```python
from build123d import *

# Parameters (mm, degrees)
SKETCH_1_W          = 100
SKETCH_1_H          = 44
EXTRUDE_1_DEPTH     = 21
CHAMFER_1_SIZE      = 5
SKETCH_2_R          = 3
CUT_EXTRUDE_1_DEPTH = 112.251966275
SKETCH_3_W          = 9
SKETCH_3_H          = 9
CUT_EXTRUDE_2_DEPTH = 9.5
SKETCH_4_R          = 18
CUT_EXTRUDE_3_DEPTH = 2
SKETCH_5_W          = 10
SKETCH_5_H          = 10
CUT_EXTRUDE_4_DEPTH = 9
FILLET_1_R          = 7


with BuildPart() as part:
    # 草图1 → 凸台-拉伸1 (new body)
    with BuildSketch(Plane(origin=(0, 0, 0), x_dir=(1, 0, 0), z_dir=(0, 1, 0))):
        with Locations((50, 22)):
            Rectangle(SKETCH_1_W, SKETCH_1_H)
    extrude(amount=EXTRUDE_1_DEPTH)

    # 倒角1
    chamfer_1_edges = [part.edges().sort_by_distance(p)[0] for p in [
        (50, 0, -44),
        (50, 0, 0),
    ]]
    chamfer(chamfer_1_edges, length=CHAMFER_1_SIZE)

    # 草图2 → 切除-拉伸1 (cut, through all)
    with BuildSketch(Plane(origin=(0, 21, 0), x_dir=(1, 0, 0), z_dir=(0, 1, 0))):
        with Locations(Location((96, 4, 0), (0, 0, 270))):
            Circle(SKETCH_2_R)
        with Locations(Location((4, 4, 0), (0, 0, 160.528779366))):
            Circle(SKETCH_2_R)
        with Locations(Location((4, 40, 0), (0, 0, 270))):
            Circle(SKETCH_2_R)
        with Locations(Location((96, 40, 0), (0, 0, 199.471220634))):
            Circle(SKETCH_2_R)
    extrude(amount=-CUT_EXTRUDE_1_DEPTH, mode=Mode.SUBTRACT)

    # 草图3 → 切除-拉伸2 (cut)
    with BuildSketch(Plane(origin=(0, 21, 0), x_dir=(1, 0, 0), z_dir=(0, 1, 0))):
        with Locations((95.5, 4.5)):
            Rectangle(SKETCH_3_W, SKETCH_3_H)
        with Locations((4.5, 4.5)):
            Rectangle(SKETCH_3_W, SKETCH_3_H)
        with Locations((95.5, 39.5)):
            Rectangle(SKETCH_3_W, SKETCH_3_H)
        with Locations((4.5, 39.5)):
            Rectangle(SKETCH_3_W, SKETCH_3_H)
    extrude(amount=-CUT_EXTRUDE_2_DEPTH, mode=Mode.SUBTRACT)

    # 草图4 → 切除-拉伸3 (cut)
    with BuildSketch(Plane(origin=(0, 21, 0), x_dir=(1, 0, 0), z_dir=(0, 1, 0))):
        with Locations(Location((28.5, 22, 0), (0, 0, 270))):
            Circle(SKETCH_4_R)
        with Locations(Location((71.5, 22, 0), (0, 0, 90))):
            Circle(SKETCH_4_R)
    extrude(amount=-CUT_EXTRUDE_3_DEPTH, mode=Mode.SUBTRACT)

    # 草图5 → 切除-拉伸4 (cut)
    with BuildSketch(Plane.XZ):
        with Locations((95, -39)):
            Rectangle(SKETCH_5_W, SKETCH_5_H)
        with Locations((95, -5)):
            Rectangle(SKETCH_5_W, SKETCH_5_H)
        with Locations((5, -5)):
            Rectangle(SKETCH_5_W, SKETCH_5_H)
        with Locations((5, -39)):
            Rectangle(SKETCH_5_W, SKETCH_5_H)
    extrude(amount=-CUT_EXTRUDE_4_DEPTH, mode=Mode.SUBTRACT)

    # 圆角1
    # the kernel refuses this fillet: 7 mm, written as the material it adds along each edge
    with BuildSketch(Plane(origin=(9, 21, -35), x_dir=(-1, 0, 0), z_dir=(0, -1, 0))) as fillet_1_piece_1:
        with BuildLine():
            CenterArc((FILLET_1_R, FILLET_1_R), FILLET_1_R, 180, 90)
            Line((0, FILLET_1_R), (0, 0))
            Line((0, 0), (FILLET_1_R, 0))
        make_face()
    extrude(amount=9.5)
    with BuildSketch(Plane(origin=(9, 21, -9), x_dir=(0, 0, 1), z_dir=(0, -1, 0))) as fillet_1_piece_2_section:
        with BuildLine():
            CenterArc((FILLET_1_R, FILLET_1_R), FILLET_1_R, 180, 90)
            Line((0, FILLET_1_R), (0, 0))
            Line((0, 0), (FILLET_1_R, 0))
        make_face()
    fillet_1_piece_2 = extrude(amount=27, mode=Mode.PRIVATE)
    fillet_1_piece_2 = split(fillet_1_piece_2, bisect_by=Plane(origin=(7.436424427, 9, -7.436424427), z_dir=(0, 1, 0)), keep=Keep.TOP, mode=Mode.PRIVATE)
    add(fillet_1_piece_2)
    with BuildSketch(Plane(origin=(10, 0, -10), x_dir=(0, 0, 1), z_dir=(0, 1, 0))) as fillet_1_piece_3_section:
        with BuildLine():
            CenterArc((FILLET_1_R, -FILLET_1_R), FILLET_1_R, 90, 90)
            Line((0, -FILLET_1_R), (0, 0))
            Line((0, 0), (FILLET_1_R, 0))
        make_face()
    fillet_1_piece_3 = extrude(amount=26.5, mode=Mode.PRIVATE)
    fillet_1_piece_3 = split(fillet_1_piece_3, bisect_by=Plane(origin=(9.565673238, 1.191688147, -3.808311853), z_dir=(0, 0.7071067811865476, -0.7071067811865476)), keep=Keep.TOP, mode=Mode.PRIVATE)
    fillet_1_piece_3 = split(fillet_1_piece_3, bisect_by=Plane(origin=(9.565673238, 21, -7.128953399), z_dir=(0, -1, 0)), keep=Keep.TOP, mode=Mode.PRIVATE)
    add(fillet_1_piece_3)
    with BuildSketch(Plane(origin=(10, 0, -34), x_dir=(-1, 0, 0), z_dir=(0, 1, 0))) as fillet_1_piece_4_section:
        with BuildLine():
            CenterArc((FILLET_1_R, -FILLET_1_R), FILLET_1_R, 90, 90)
            Line((0, -FILLET_1_R), (0, 0))
            Line((0, 0), (FILLET_1_R, 0))
        make_face()
    fillet_1_piece_4 = extrude(amount=26.5, mode=Mode.PRIVATE)
    fillet_1_piece_4 = split(fillet_1_piece_4, bisect_by=Plane(origin=(7.120179523, 21, -34.433198562), z_dir=(0, -1, 0)), keep=Keep.TOP, mode=Mode.PRIVATE)
    fillet_1_piece_4 = split(fillet_1_piece_4, bisect_by=Plane(origin=(7.120179523, -0.033400719, -38.966599281), z_dir=(0, 0.7071067811865476, 0.7071067811865476)), keep=Keep.TOP, mode=Mode.PRIVATE)
    add(fillet_1_piece_4)
    with BuildSketch(Plane(origin=(91, 21, -35), x_dir=(1, 0, 0), z_dir=(0, -1, 0)), Plane(origin=(91, 21, -9), x_dir=(0, 0, 1), z_dir=(0, -1, 0))) as fillet_1_piece_5:
        with BuildLine():
            CenterArc((FILLET_1_R, -FILLET_1_R), FILLET_1_R, 90, 90)
            Line((0, -FILLET_1_R), (0, 0))
            Line((0, 0), (FILLET_1_R, 0))
        make_face()
    extrude(amount=9.5)
    with BuildSketch(Plane(origin=(90, 0, -34), x_dir=(1, 0, 0), z_dir=(0, 1, 0))) as fillet_1_piece_6_section:
        with BuildLine():
            CenterArc((FILLET_1_R, FILLET_1_R), FILLET_1_R, 180, 90)
            Line((0, FILLET_1_R), (0, 0))
            Line((0, 0), (FILLET_1_R, 0))
        make_face()
    fillet_1_piece_6 = extrude(amount=26.5, mode=Mode.PRIVATE)
    fillet_1_piece_6 = split(fillet_1_piece_6, bisect_by=Plane(origin=(92.879820477, 21, -34.433198562), z_dir=(0, -1, 0)), keep=Keep.TOP, mode=Mode.PRIVATE)
    fillet_1_piece_6 = split(fillet_1_piece_6, bisect_by=Plane(origin=(92.879820477, -0.033400719, -38.966599281), z_dir=(0, 0.7071067811865476, 0.7071067811865476)), keep=Keep.TOP, mode=Mode.PRIVATE)
    add(fillet_1_piece_6)
    with BuildSketch(Plane(origin=(90, 0, -10), x_dir=(0, 0, 1), z_dir=(0, 1, 0))) as fillet_1_piece_7_section:
        with BuildLine():
            CenterArc((FILLET_1_R, FILLET_1_R), FILLET_1_R, 180, 90)
            Line((0, FILLET_1_R), (0, 0))
            Line((0, 0), (FILLET_1_R, 0))
        make_face()
    fillet_1_piece_7 = extrude(amount=26.5, mode=Mode.PRIVATE)
    fillet_1_piece_7 = split(fillet_1_piece_7, bisect_by=Plane(origin=(90.434326762, 1.191688147, -3.808311853), z_dir=(0, 0.7071067811865476, -0.7071067811865476)), keep=Keep.TOP, mode=Mode.PRIVATE)
    fillet_1_piece_7 = split(fillet_1_piece_7, bisect_by=Plane(origin=(90.434326762, 21, -7.128953399), z_dir=(0, -1, 0)), keep=Keep.TOP, mode=Mode.PRIVATE)
    add(fillet_1_piece_7)


solid = part.part
```
Read the model definition and answer for the solid it produces. Units are mm, in the model's axes. A direction names the side the tool comes from. Give positions to 0.01 mm unless a question says otherwise; leave off trailing zeros. Order: outer loops, then holes, each group sorted by start corner. A loop starts at its lowest first (then second) coordinate and runs counter-clockwise, first axis right, second up.
(1) For faces 1 (the flat face through (1, 16, -35)), 2 (the flat face through (93, 9, -5)), 3 (the flat face through (5, 9, -7)), 4 (the cylindrical face through (92, 4.4, -36.1)), 5 (the flat face through (99, 16, -9)), determine the directions among +Z, -Z, +X, -X, +Y, -Y from which every point of the face is accessible in a straight line to the end or side of a thin tool.
(2) Given pin 1 (0.6 mm diameter, centred on y = 14, z = -42.5, fed in from -X); pin 2 (7 mm diameter, centred on x = 97, z = -3.5, fed in from +Y); pin 3 (0.9 mm diameter, centred on y = 7, z = -2, fed in from +X), each flat-ended and moving along its own axis, determine where each tip first touches the part or whether it passes through.
(3) Find section D-D (x = 96). Give the vertices of the cut face in (y, z).
(4) Find section B-B (x = 28.5). Give the vertices of the cut face in (y, z), plus the area to 3 significant figures.
(5) For a pull along Z with two mould halves and no side action, classify faces 6 (the flat face through (29, 19, -22)), 7 (the flat face through (1, 4, -34)), 8 (the flat face through (10, 6, -43)) as released by +Z, released by -Z, zero draft, split by the parting line, or undercut.
(6) Straight lines are drawn through the part: L1, parallel to X at y = 10.45, z = -4; L2, parallel to X at y = 19.55, z = -22; L3, parallel to Z at x = 71.5, y = 20.15. For each, find the intervals that lie inside material, in ascending order.
(7) Find section A-A (z = -22). Give the vertices of the cut face in (x, y).
(8) Find section C-C (y = 6). Give the vertices of the cut face in (x, z), plus the area to 3 significant figures.
Result sheet:
1. face 1: -Z, -X, +Y
1. face 2: +Z, +X, -Y
1. face 3: +Z, -X, -Y
1. face 4: -Z, +X, -Y
1. face 5: +Z, +X, +Y
2. pin 1: stops at x = 9
2. pin 2: stops at y = 11.5
2. pin 3: stops at x = 90
3. outline: (0, -34.07) - (9, -34.07) - (9, -37) - (11.5, -37) - (11.5, -35.29) - (21, -35.29) - (21, -8.71) - (11.5, -8.71) - (11.5, -7) - (9, -7) - (9, -9.93) - (0, -9.93) - close; (9, -44) - (11.5, -44) - (11.5, -43) - (9, -43) - close; (9, -1) - (11.5, -1) - (11.5, 0) - (9, 0) - close
4. outline: (0, -39) - (5, -44) - (21, -44) - (21, -40) - (19, -40) - (19, -4) - (21, -4) - (21, 0) - (5, 0) - (0, -5) - close
4. area: 827 mm2
5. face 6: undercut
5. face 7: released by -Z
5. face 8: zero draft
6. L1: x = 0 to 1, 7 to 93, 99 to 100
6. L2: x = 0 to 10.5, 46.5 to 53.5, 89.5 to 100
6. L3: z = -44 to -40, -4 to 0
7. outline: (0, 0) - (100, 0) - (100, 21) - (89.5, 21) - (89.5, 19) - (53.5, 19) - (53.5, 21) - (46.5, 21) - (46.5, 19) - (10.5, 19) - (10.5, 21) - (0, 21) - close
8. outline: (0, -34) - (3, -34) arc R7 cw to (10, -41) - (10, -44) - (90, -44) - (90, -41) arc R7 cw to (97, -34) - (100, -34) - (100, -10) - (97, -10) arc R7 cw to (90, -3) - (90, 0) - (10, 0) - (10, -3) arc R7 cw to (3, -10) - (0, -10) - close
8. area: 4,040 mm2
